The figure shows three views and two pictorial views of one solid part (mm, origin at its lowest corner). Answer the questions. A direction names the side the tool comes from. Give positions to 0.01 mm unless a question says otherwise; leave off trailing zeros. Order: outer loops, then holes, each group sorted by start corner. A loop starts at its lowest first (then second) coordinate and runs counter-clockwise, first axis right, second up. Notation, with made-up numbers: M 39.25,-25 L 60.25,-25 A20 ccw 60.25,-14 Z; hole C 16.5,25 d9. An arc over 180 degrees is marked long. One line per item, written item: value.
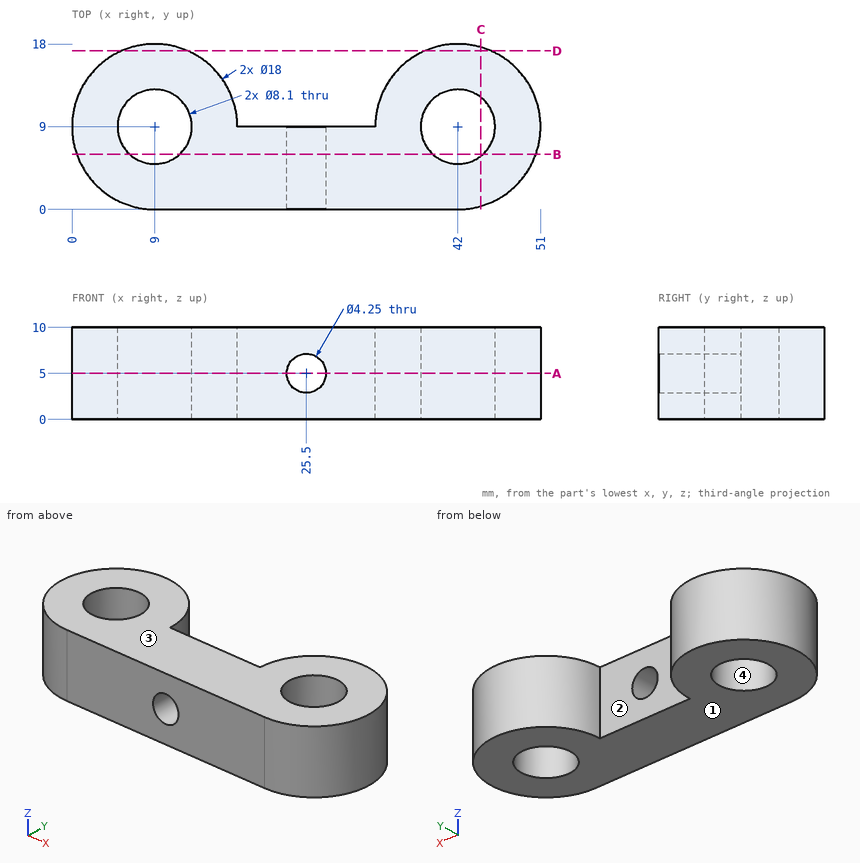
1) This flat-tipped pin is pushed along its axis until it touches: pin 1 Ø1 at (y, z) = (3.5, 3) entering from +X. Where does it stop, or does it pass through?
Reported:
pin 1: stops at x = 49.48
2) Which of the six approach directions +Z, -Z, +X, -X, +Y, -Y give full straight-line access (tool end or side, diameter ignored) to the marked faces 1 and 2?
Reported:
face 1: -Z, +X, -X, +Y, -Y
face 2: +Z, -Z, +Y
3) Consider probe 1 along X at (y, z) = (10.5, 6); probe 2 along Z at (x, y) = (25.5, 7) (3 decimals); probe 3 along X at (y, z) = (12.5, 2.5). Determine where each line is inside the solid, lowest interval first.
Reported:
probe 1: x = 0.13 to 5.24, 12.76 to 17.87, 33.13 to 38.24, 45.76 to 50.87
probe 2: z = 0 to 2.875, 7.125 to 10
probe 3: x = 0.71 to 6.96, 11.04 to 17.29, 33.71 to 39.96, 44.04 to 50.29
4) Find section B-B, the plane y = 6. Write down the section's boundary in (x, z) (3 decimals), plus the area to 3 significant figures.
Reported:
outline: M 0.515,0 L 6.279,0 L 6.279,10 L 0.515,10 Z; M 11.721,0 L 39.279,0 L 39.279,10 L 11.721,10 Z; M 44.721,0 L 50.485,0 L 50.485,10 L 44.721,10 Z; hole C 25.5,5 d4.25
area: 377 mm^2
5) Find section C-C, the plane x = 44.5. Write down the section's boundary in (y, z), plus the area to 3 significant figures.
Reported:
outline: M 0.35,0 L 5.81,0 L 5.81,10 L 0.35,10 Z; M 12.19,0 L 17.65,0 L 17.65,10 L 12.19,10 Z
area: 109 mm^2
6) Find section D-D, the plane y = 17.25. Write down the section's boundary in (x, z).
Reported:
outline: M 5.4,0 L 12.6,0 L 12.6,10 L 5.4,10 Z; M 38.4,0 L 45.6,0 L 45.6,10 L 38.4,10 Z
7) Determine the mould class of the marked faces 3 and 4 for opening direction X: +X half, -X half, draft (parallel to the pull), parting line (faces both ways), or undercut.
Reported:
face 3: draft
face 4: undercut
8) Find section A-A, the plane z = 5. Write down the section's boundary in (x, y) (3 decimals).
Reported:
outline: M 9,0 L 23.375,0 L 23.375,9 L 18,9 A9 ccw long Z; M 27.625,0 L 42,0 A9 ccw long 33,9 L 27.625,9 Z; hole C 9,9 d8.1; hole C 42,9 d8.1
